Model file for the job. Use its own axes, mm. A direction names the side the tool comes from. Round coordinates to 2 decimals unless told otherwise and drop trailing zeros. Order: outer loops, then holes, each group sorted by start corner. A loop starts at its lowest first (then second) coordinate and runs counter-clockwise, first axis right, second up. Notation, with made-up numbers: M 40,-24 L 93,-24 A29 ccw 93,2 Z; hole C 9.5,4 d6. An arc over 180 degrees is marked long. Return JSON: item names as keys, results as strings. Group by question number.
Item 1: Which spindle directions (+Z, -Z, +X, -X, +Y, -Y) get a long thin tool onto all of the face, cutting with end or side? Do faces 1 (the face through (213, 7.5, -20)), 2 (the face through (213, 2.5, -20)), 3 (the face through (7, 7.5, -20)), 4 (the face through (213, 5, -2.5)), 5 (the face through (7, 5, -37.5)). Say none if no direction does.
Item 2: Pin check, flat tips, straight feed: pin 1 Ø4 at (x, y) = (8, 4.5) entering from +Z; pin 2 Ø2.5 at (x, y) = (211, 5) entering from -Z; pin 3 Ø7.5 at (x, z) = (4.5, -19) entering from +Y. Stop position of each tip, or through.
Item 3: Slice it at C-C on y = 5.75. Write the cut outline in (x, z).
Item 4: Probe line 1 along Z through (x, y) = (110.5, 7); line 2 along X through (y, z) = (7, -20); line 3 along X through (y, z) = (0.75, -20). List the from-to ranges inside material, lowest first.
from build123d import *

# Parameters (mm, degrees)
ESBO_O1_W                  = 220
ESBO_O1_H                  = 40
RESSALTO_EXTRUS_O1_DEPTH   = 10
ESBO_O2_W                  = 40
ESBO_O2_H                  = 10
ESBO_O2_W_2                = 35
ESBO_O2_H_2                = 5
CORTE_EXTRUS_O1_DEPTH      = 15
CORTE_EXTRUS_O2_DEPTH      = 224.830292856
CORTE_EXTRUS_O2_DEPTH_BACK = 224.830292856
ESBO_O3_R                  = 14.5
CORTE_EXTRUS_O3_DEPTH      = 224.830292856
CORTE_EXTRUS_O3_DEPTH_BACK = 8.5
ESBO_O4_R                  = 16
ESBO_O4_R_2                = 14.5
FILETE1_R                  = 1.5


with BuildPart() as part:
    # Esboço1 → Ressalto-extrusão1 (new body)
    with BuildSketch(Plane(origin=(0, 0, 0), x_dir=(1, 0, 0), z_dir=(0, 1, 0))):
        with Locations((110, 20)):
            Rectangle(ESBO_O1_W, ESBO_O1_H)
    extrude(amount=RESSALTO_EXTRUS_O1_DEPTH)

    # Esboço2 → Corte-extrusão1 (cut)
    with BuildSketch(Plane.ZY):
        with Locations((-20, 5)):
            Rectangle(ESBO_O2_W, ESBO_O2_H)
        with Locations((-20, 5)):
            Rectangle(ESBO_O2_W_2, ESBO_O2_H_2, mode=Mode.SUBTRACT)
    corte_extrus_o1 = extrude(amount=-CORTE_EXTRUS_O1_DEPTH, mode=Mode.SUBTRACT)

    # Espelhar1: Corte-extrusão1 across plane
    add(corte_extrus_o1.mirror(Plane.ZY.offset(-110)), mode=Mode.SUBTRACT)

    # Esboço3 → Corte-extrusão2 (cut, two sides: drawn at the far end of the back side and taken through both)
    with BuildSketch(Plane(origin=(0, 0, 0), x_dir=(1, 0, 0), z_dir=(0, 1, 0)).offset(-CORTE_EXTRUS_O2_DEPTH_BACK)):
        with Locations(Location((110, 20, 0), (0, 0, 270))):
            Circle(ESBO_O3_R)
    extrude(amount=CORTE_EXTRUS_O2_DEPTH + CORTE_EXTRUS_O2_DEPTH_BACK, mode=Mode.SUBTRACT)

    # Esboço4 → Corte-extrusão3 (cut, two sides: drawn at the far end of the back side and taken through both)
    with BuildSketch(Plane(origin=(0, 10, 0), x_dir=(1, 0, 0), z_dir=(0, 1, 0)).offset(-CORTE_EXTRUS_O3_DEPTH_BACK)):
        with Locations(Location((110, 20, 0), (0, 0, 90))):
            Circle(ESBO_O4_R)
        with Locations(Location((110, 20, 0), (0, 0, 270))):
            Circle(ESBO_O4_R_2, mode=Mode.SUBTRACT)
    extrude(amount=CORTE_EXTRUS_O3_DEPTH + CORTE_EXTRUS_O3_DEPTH_BACK, mode=Mode.SUBTRACT)

    # Filete1
    filete1_edges = [part.edges().sort_by_distance(p)[0] for p in [
        (110, 1.5, -4),
    ]]
    fillet(filete1_edges, radius=FILETE1_R - 0.0001)  # a hair under: the kernel refuses the full size


solid = part.part
Output values:
{
 "1": {"face 1": "+Z, -Z, +X, +Y", "face 2": "+Z, -Z, +X, -Y", "face 3": "+Z, -Z, -X, +Y", "face 4": "+Z, +X, +Y, -Y", "face 5": "-Z, -X, +Y, -Y"},
 "2": {"pin 1": "z = -2.5", "pin 2": "z = -37.5", "pin 3": "y = 7.5"},
 "3": {"outline": "M 0,-37.5 L 15,-37.5 L 15,-40 L 205,-40 L 205,-37.5 L 220,-37.5 L 220,-2.5 L 205,-2.5 L 205,0 L 15,0 L 15,-2.5 L 0,-2.5 Z; hole C 110,-20 d32"},
 "4": {"line 1": "-40 to -35.99, -4.01 to 0", "line 2": "0 to 94, 126 to 220", "line 3": "15 to 95.5, 124.5 to 205"}
}
